from build123d import *

# Parameters (mm, degrees)
F1_DEPTH = 63.5
F0_W     = 18.0850151875
F0_H     = 19.05
F2_DEPTH = 25.4
F3_DEPTH = 7.9375
F5_R     = 5.08
F6_R     = 5.08


with BuildPart() as f1:
    # F0 (on Front) → F1 (new body, symmetric)
    with BuildSketch(Plane.XZ):
        Polygon((-41.275, -9.525), (41.275, -9.525), (41.275, 9.525), (22.225, 9.525), (-41.275, 9.525), align=None)
    extrude(amount=F1_DEPTH, both=True)

    # F0 (on Front) → F2 (join, symmetric)
    with BuildSketch(Plane.XZ):
        with BuildLine():
            Line((22.225, 9.525), (41.275, 9.525))
            Line((41.275, 9.525), (41.275, 27.0002))
            ThreePointArc((41.275, 27.0002), (45.9246798487, 38.2255201513), (57.15, 42.8752))
            Line((57.15, 42.8752), (60.325, 42.8752))
            Line((60.325, 42.8752), (60.325, 61.9252))
            Line((60.325, 61.9252), (57.15, 61.9252))
            ThreePointArc((57.15, 61.9252), (32.4542956671, 51.6959043329), (22.225, 27.0002))
            Line((22.225, 27.0002), (22.225, 9.525))
        make_face()
        with Locations((69.3675075937, 52.4002)):
            Rectangle(F0_W, F0_H)
    extrude(amount=F2_DEPTH, both=True)

    # F0 (on Front) → F3 (join, symmetric)
    with BuildSketch(Plane.XZ):
        with BuildLine():
            add(Edge.make_bspline(
                [(-41.275, 9.525), (-37.5866588905, 18.8099618573), (-19.5091748913, 37.7919660038), (11.8441398709, 58.454694521), (42.3775529044, 62.5964135267), (57.15, 61.9252)],
                knots=[0, 0, 0, 0, 0.3130865631, 0.6429480461, 1, 1, 1, 1], degree=3))
            Line((-41.275, 9.525), (22.225, 9.525))
            Line((22.225, 9.525), (22.225, 27.0002))
            ThreePointArc((22.225, 27.0002), (32.4542956671, 51.6959043329), (57.15, 61.9252))
        make_face()
    extrude(amount=F3_DEPTH, both=True)

    # F0 (on Front) → F4 (revolve)
    with BuildSketch(Plane.XZ):
        Polygon((78.4100151875, 66.675), (78.4100151875, 61.9252), (78.4100151875, 42.8752), (78.4100151875, 38.1), (111.125, 38.1), (111.125, 66.675), align=None)
    revolve(axis=Axis((78.4100151875, 0, 52.3875), (0, 0, -1)))

    # F5
    f5_edges = [f1.edges().sort_by_distance(p)[0] for p in [
        (-41.275, -63.5, 0),
        (41.275, -63.5, 0),
    ]]
    fillet(f5_edges, radius=F5_R)

    # F6
    f6_edges = [f1.edges().sort_by_distance(p)[0] for p in [
        (41.275, 63.5, 0),
        (-41.275, 63.5, 0),
    ]]
    fillet(f6_edges, radius=F6_R)


solid = f1.part
Here's how the part is built. I have some questions about the finished solid (model axes, mm). A direction names the side the tool comes from. Coordinates: 2 decimals unless noted, no trailing zeros. Write each loop counter-clockwise with the first axis right and the second up, starting at its lowest first coordinate (ties: lowest second). Pieces come first, ordered by that corner, then holes.
1) If we section it at D-D (y = -23): List the corners of the cut face in (x, z) for me (3 decimals).
Filled in:
outline: (-41.275, -9.525) - (41.275, -9.525) - (41.275, 27) arc R15.875 cw to (55.145, 42.748) - (55.145, 38.1) - (101.675, 38.1) - (101.675, 66.675) - (55.145, 66.675) - (55.145, 61.868) arc R34.925 ccw to (22.225, 27) - (22.225, 9.525) - (-41.275, 9.525) - close
2) If we section it at B-B (y = 19): List the corners of the cut face in (x, z) for me (3 decimals), plus the area to 3 significant figures.
Filled in:
outline: (-41.275, -9.525) - (41.275, -9.525) - (41.275, 27) arc R15.875 cw to (51.778, 41.939) - (51.778, 38.1) - (105.042, 38.1) - (105.042, 66.675) - (51.778, 66.675) - (51.778, 61.51) arc R34.925 ccw to (22.225, 27) - (22.225, 9.525) - (-41.275, 9.525) - close
area: 4,080 mm2
3) If we section it at C-C (x = 81): List the corners of the cut face in (y, z) for me (3 decimals).
Filled in:
outline: (-32.612, 38.1) - (32.612, 38.1) - (32.612, 66.675) - (-32.612, 66.675) - close
4) I'm going to push flat-ended pins straight in: pin 1 (5 mm diameter, centred on y = 21, z = 14, fed in from -X) (3 decimals); pin 2 (1 mm diameter, centred on x = 3.5, z = 14.5, fed in from +Y); pin 3 (3 mm diameter, centred on y = -25.5, z = 45, fed in from -X). Where does each tip first touch, or does it pass through?
Filled in:
pin 1: stops at x = 22.225
pin 2: stops at y = 7.94
pin 3: stops at x = 26.37
5) Which directions (+Z, -Z, +X, -X, +Y, -Y) give clear straight access to the entire face, cutting with the end or side of a thin tool? Please do faces 1 (the face through (28.763, 16.547, 47.346)), 2 (the face through (-1, 63.5, 0)), 3 (the face through (79, 0, 38.1)), 4 (the face through (3, -7.938, 30)).
Filled in:
face 1: +Z, -X, +Y
face 2: +Z, -Z, +X, -X, +Y
face 3: -Z, +X, +Y, -Y
face 4: +Z, -X, -Y
6) If I drill on line 1 (Y direction, x = -17.5, z = 35); line 2 (Y direction, x = 44, z = 37.5); line 3 (X direction, y = 1, z = 1.5) (3 decimals), over which ranges is the centre line in solid material (lowest first)?
Filled in:
line 1: y = -7.94 to 7.94
line 2: y = -25.4 to 25.4
line 3: x = -41.275 to 41.275
7) If we section it at A-A (z = 3.5): List the corners of the cut face in (x, y) for me (3 decimals), plus the area to 3 significant figures.
Filled in:
outline: (-41.275, -58.42) arc R5.08 ccw to (-36.195, -63.5) - (36.195, -63.5) arc R5.08 ccw to (41.275, -58.42) - (41.275, 58.42) arc R5.08 ccw to (36.195, 63.5) - (-36.195, 63.5) arc R5.08 ccw to (-41.275, 58.42) - close
area: 10,500 mm2
